from build123d import *

# Parameters (mm, degrees)
SKETCH1_W                      = 23.5
SKETCH1_H                      = 28.25
BASE_FLANGE1_DEPTH             = 1.5
EDGE_FLANGE1_STRIP_W           = 10
EDGE_FLANGE1_STRIP_H           = 1.5
EDGE_FLANGE1_STRIP_CUT_DEPTH   = 28.25
EDGE_FLANGE1_STRIP_2_W         = 10
EDGE_FLANGE1_STRIP_2_H         = 1.5
EDGE_FLANGE1_STRIP_CUT_2_DEPTH = 28.25
EDGE_FLANGE1_DEPTH             = 28.25
EDGE_FLANGE1_BEND_DEPTH        = 28.25
SKETCH12_R                     = 1.6
SKETCH12_R_2                   = 4.75
CUT_EXTRUDE1_DEPTH             = 26.12126838
SKETCH13_R                     = 1.1
SKETCH13_W                     = 29.65
SKETCH13_H                     = 20
CUT_EXTRUDE2_DEPTH             = 35.025955167
FILLET1_R                      = 1.25
FILLET2_R                      = 1


# Sheet-metal steps are written as plain solids
with BuildPart() as part:
    # Sketch1 → Base-Flange1 (new body)
    with BuildSketch(Plane.XY):
        Rectangle(SKETCH1_W, SKETCH1_H)
    extrude(amount=-BASE_FLANGE1_DEPTH)

    # Edge-Flange1 strip (across the edge) → Edge-Flange1 strip cut (cut)
    with BuildSketch(Plane(origin=(11.75, 14.125, -1.5), x_dir=(-1, 0, 0), z_dir=(0, -1, 0))):
        with Locations((-3, -0.75)):
            Rectangle(EDGE_FLANGE1_STRIP_W, EDGE_FLANGE1_STRIP_H)
    extrude(amount=EDGE_FLANGE1_STRIP_CUT_DEPTH, mode=Mode.SUBTRACT)

    # Edge-Flange1 strip 2 (across the edge) → Edge-Flange1 strip cut 2 (cut)
    with BuildSketch(Plane(origin=(-11.75, -14.125, -1.5), x_dir=(1, 0, 0), z_dir=(0, 1, 0))):
        with Locations((-3, -0.75)):
            Rectangle(EDGE_FLANGE1_STRIP_2_W, EDGE_FLANGE1_STRIP_2_H)
    extrude(amount=EDGE_FLANGE1_STRIP_CUT_2_DEPTH, mode=Mode.SUBTRACT)

    # Edge-Flange1 section (across the edge) → Edge-Flange1 (add)
    with BuildSketch(Plane(origin=(11.75, 14.125, -1.5), x_dir=(-1, 0, 0), z_dir=(0, -1, 0))):
        with BuildLine():
            Line((-1.5, 2), (-1.5, 14.5))
            Line((-1.5, 14.5), (0, 14.5))
            Line((0, 14.5), (0, 2))
            ThreePointArc((0, 2), (0.585786438, 0.585786438), (2, 0))
            Line((2, 0), (2, -1.5))
            ThreePointArc((2, -1.5), (-0.474873734, -0.474873734), (-1.5, 2))
        make_face()
    extrude(amount=EDGE_FLANGE1_DEPTH)

    # Edge-Flange1 section 2 (across the edge) → Edge-Flange1 bend (add)
    with BuildSketch(Plane(origin=(-11.75, -14.125, -1.5), x_dir=(1, 0, 0), z_dir=(0, 1, 0))):
        with BuildLine():
            Line((-1.5, 2), (-1.5, 14.5))
            Line((-1.5, 14.5), (0, 14.5))
            Line((0, 14.5), (0, 2))
            ThreePointArc((0, 2), (0.585786438, 0.585786438), (2, 0))
            Line((2, 0), (2, -1.5))
            ThreePointArc((2, -1.5), (-0.474873734, -0.474873734), (-1.5, 2))
        make_face()
    extrude(amount=EDGE_FLANGE1_BEND_DEPTH)

    # Sketch12 → Cut-Extrude1 (cut, through all)
    with BuildSketch(Plane.XY):
        with Locations((-6, 6)):
            Circle(SKETCH12_R)
        with Locations((6, 6)):
            Circle(SKETCH12_R)
        with Locations((6, -6)):
            Circle(SKETCH12_R)
        with Locations((-6, -6)):
            Circle(SKETCH12_R)
        Circle(SKETCH12_R_2)
    extrude(amount=-CUT_EXTRUDE1_DEPTH, mode=Mode.SUBTRACT)

    # Sketch13 → Cut-Extrude2 (cut, through all)
    with BuildSketch(Plane(origin=(13.25, 0, 0), x_dir=(0, 0, -1), z_dir=(1, 0, 0))):
        with Locations((13.6, 11.525)):
            Circle(SKETCH13_R)
        with Locations((13.6, -11.525)):
            Circle(SKETCH13_R)
        with Locations((25.125, 0)):
            Rectangle(SKETCH13_W, SKETCH13_H)
    extrude(amount=-CUT_EXTRUDE2_DEPTH, mode=Mode.SUBTRACT)

    # Fillet1
    fillet1_edges = [part.edges().sort_by_distance(p)[0] for p in [
        (12.5, -10, -10.3),
        (12.5, 10, -10.3),
        (-12.5, -10, -10.3),
        (-12.5, 10, -10.3),
    ]]
    fillet(fillet1_edges, radius=FILLET1_R)

    # Fillet2
    fillet2_edges = [part.edges().sort_by_distance(p)[0] for p in [
        (-12.5, 10, -16),
        (-12.5, -10, -16),
        (12.5, -10, -16),
        (12.5, 10, -16),
        (12.5, 14.125, -16),
        (12.5, -14.125, -16),
        (-12.5, -14.125, -16),
        (-12.5, 14.125, -16),
    ]]
    fillet(fillet2_edges, radius=FILLET2_R)


solid = part.part
Here's how the part is built. I have some questions about the finished solid (model axes, mm). A direction names the side the tool comes from. Coordinates: 2 decimals unless noted, no trailing zeros. Write each loop counter-clockwise with the first axis right and the second up, starting at its lowest first coordinate (ties: lowest second). Pieces come first, ordered by that corner, then holes. Notation, with made-up numbers: (69.25, 11.25) - (106.25, 11.25) arc R26 ccw to (106.25, 39.25) - close; hole circle Ø4 at (83, 25.25). An arc over 180 degrees is marked (long way). Use one line per item in the form item = value.
1) On a 3-axis mill with a long thin cutter (end or side, diameter ignored), from which of +Z, -Z, +X, -X, +Y, -Y can I reach the whole of each face in a straight line? I mean faces 4 (the cylindrical face through (12.51, 12.27, -12.79)), 5 (the flat face through (4, 3, -1.5)), 6 (the flat face through (13, -10, -13)). Say none if no direction works.
Solved:
face_4 = +X, -X
face_5 = -Z, +Y, -Y
face_6 = -Z, +X, -X
2) Suppose I cut it at C-C, the plane y = 0. Write out the boundary of the cut face in (x, z), plus the area to 3 significant figures.
Solved:
outline = (-13.25, -10.3) - (-11.75, -10.3) - (-11.75, -3.5) arc R2 cw to (-9.75, -1.5) - (-4.75, -1.5) - (-4.75, 0) - (-9.75, 0) arc R3.5 ccw to (-13.25, -3.5) - close; (4.75, -1.5) - (9.75, -1.5) arc R2 cw to (11.75, -3.5) - (11.75, -10.3) - (13.25, -10.3) - (13.25, -3.5) arc R3.5 ccw to (9.75, 0) - (4.75, 0) - close
area = 48.4 mm2
3) Thinking about a two-plate mould opening in Z: for faces 1 (the cylindrical face through (12.51, -12.5, -14.11)), 2 (the cylindrical face through (6.74, 4.58, -0.74)), 3 (the cylindrical face through (-12.2, -0.2, -1)), which applies, released by +Z, released by -Z, zero draft, split by the parting line, or undercut?
Solved:
face_1 = undercut
face_2 = zero draft
face_3 = released by +Z
4) I need wall thicknesses on line 1 (Y direction, x = 12.8, z = -13.6) (3 decimals); line 2 (X direction, y = 3, z = -7.75); line 3 (Y direction, x = 6, z = -0.35) (3 decimals). Which ranges of each line are inside material? Lowest first, please.
Solved:
line_1 = -14.125 to -12.625, -10.425 to -10, 10 to 10.425, 12.625 to 14.125
line_2 = -13.25 to -11.75, 11.75 to 13.25
line_3 = -14.125 to -7.6, -4.4 to 4.4, 7.6 to 14.125
5) I'm going to push flat-ended pins straight in: P1, Ø0.8, axis at x = -12.5, y = -3, coming from the -Z side; P2, Ø4, axis at x = 6, y = -6, coming from the -Z side. Where does each tip first touch, or does it pass through?
Solved:
P1 = -10.3
P2 = -1.5
6) Suppose I cut it at B-B, the plane x = 6. Write out the boundary of the cut face in (y, z) (3 decimals), plus the area to 3 significant figures.
Solved:
outline = (-14.125, -1.5) - (-7.6, -1.5) - (-7.6, 0) - (-14.125, 0) - close; (-4.4, -1.5) - (4.4, -1.5) - (4.4, 0) - (-4.4, 0) - close; (7.6, -1.5) - (14.125, -1.5) - (14.125, 0) - (7.6, 0) - close
area = 32.8 mm2
7) Suppose I cut it at A-A, the plane z = -13.6. Give the number of separate pieces and of enclosed holes in the cut face, plus the area to 4 significant figures.
Solved:
separate_pieces = 8
enclosed_holes = 0
area = 11.55 mm2
8) Suppose I cut it at D-D, the plane z = -5.5. Write out the boundary of the cut face in (x, y) (3 decimals).
Solved:
outline = (-13.25, -14.125) - (-11.75, -14.125) - (-11.75, 14.125) - (-13.25, 14.125) - close; (11.75, -14.125) - (13.25, -14.125) - (13.25, 14.125) - (11.75, 14.125) - close
